Input: part model. Units: mm. Frame: model coordinates. A direction names the side the tool comes from. Coordinates: 2 decimals unless noted, no trailing zeros. Loops run counter-clockwise (first coordinate to the right, second up) from the corner with the lowest first, then second, coordinate; pieces in that order, holes last. Notation, with made-up numbers: M -20.75,8.5 L 0.25,8.5 A4 cw 0.25,15.5 Z; hole C 35.25,-12 d11. An arc over 180 degrees is marked long. Use a Markdown table: item, result. Add a question column.
1. Section B-B on z = 42.5. Output: boundary loops of the cut face in (x, y), then the cut area to 3 significant figures.
2. Section D-D on y = 7.5. Output: boundary loops of the cut face in (x, z), then the cut area to 3 significant figures.
3. Line query: L1, parallel to Z at x = -6, y = 50; L2, parallel to Y at x = -7, z = 38; L3, parallel to Y at x = -0.4, z = 38. Output: solid intervals per line, ascending. Write a range as [from, to].
4. Section C-C on x = 57. Output: boundary loops of the cut face in (y, z), then the cut area to 3 significant figures.
5. Draft query along Y for faces 1 (the cylindrical face through (-0.355, 68.506, 36.693)), 2 (the cylindrical face through (-7.145, 52.706, 39.407)), 3 (the flat face through (33, -4, 25)), 4 (the flat face through (75, 50, 1)). Return one class per face: +Y half, -Y half, draft (parallel to the pull), parting line (faces both ways), or undercut.
6. Set-up query: faces 5 (the flat face through (-4, 62.936, 13)), 6 (the flat face through (0, 49, 31)), 7 (the flat face through (-0.7, 60.4, 38)), 8 (the cylindrical face through (-7.15, 32.14, 35.85)). Return all of +Z, -Z, +X, -X, +Y, -Y with unobstructed straight access to the full face (end or side cutting, diameter ignored); none if empty.
7. Section A-A on z = 11.5. Output: boundary loops of the cut face in (x, y).
8. Pin query (flat end, axial travel): pin 1 (3 mm diameter, centred on y = 50.5, z = 38, fed in from +X); pin 2 (5 mm diameter, centred on x = 55.5, y = 37, fed in from +Z); pin 3 (8 mm diameter, centred on y = 42.1, z = 38.03, fed in from +X); pin 4 (3 mm diameter, centred on y = 58, z = 39, fed in from +X). Return the tip coordinate at first contact, or that it passes through.
Autodesk Fusion 360 part; units mm, degrees
sketch "Sketch1" plane through (0, 0, 0) normal (0, 0, 1) x (1, 0, 0)
  line L0 (0, 0) -> (140, 0)
  line L1 (140, 0) -> (140, 150)
  line L2 (140, 150) -> (0, 150)
  line L3 (0, 150) -> (0, 0)
sketch "Sketch2" plane through (0, 0, 0) normal (0, 0, 1) x (1, 0, 0)
sketch "Sketch3" plane through (0, 0, 0) normal (0, 0, 1) x (1, 0, 0)
  line L0 (0, 0) -> (0, 100)
  line L1 (0, 100) -> (75, 100)
  line L2 (75, 100) -> (75, 0)
  line L3 (75, 0) -> (0, 0)
  line L4 (75, 100) -> (75, 104)
  line L5 (75, 104) -> (-7.5, 104)
  line L6 (-7.5, 104) -> (-7.5, -4)
  line L7 (-7.5, -4) -> (75, -4)
  line L8 (75, -4) -> (75, 0)
  dimension "d4" = 75
  dimension "d5" = 4
  dimension "d6" = 82.5
  dimension "d7" = 108
  dimension "d8" = 82.5
extrude "Extrude2" add sketch "Sketch3" along normal blind 50 contours L0 L1 L3 L4 L5 L6 L7 L8
sketch "Sketch4" plane through (0, 0, 0) normal (0, 0, 1) x (1, 0, 0)
sketch "Sketch5" plane through (0, 0, 0) normal (0, 0, 1) x (1, 0, 0)
  line L0 (75, 0) -> (75, 100)
  line L1 (75, 100) -> (0, 100)
  line L2 (0, 100) -> (0, 0)
  line L3 (0, 0) -> (75, 0)
extrude "Extrude3" add sketch "Sketch5" along normal blind 1.2
sketch "Sketch6" plane through (0, 0, 0) normal (1, 0, 0) x (0, 1, 0)
  line L0 (0, 1.2) -> (100, 1.2)
  line L1 (100, 1.2) -> (100, 50)
  line L2 (100, 50) -> (0, 50)
  line L3 (0, 50) -> (0, 1.2)
sketch "Sketch7" plane through (0, 0, 0) normal (1, 0, 0) x (0, 1, 0)
  line L0 (92, -12) -> (91.9892, -11.1216)
sketch "Sketch8" plane through (0, 0, 0) normal (1, 0, 0) x (0, 1, 0)
sketch "Sketch9" plane through (0, 0, 0) normal (1, 0, 0) x (0, 1, 0)
sketch "Sketch10" plane through (0, 0, 0) normal (1, 0, 0) x (0, 1, 0)
  line L0 (0, 1.2) -> (100, 1.2)
  line L1 (100, 1.2) -> (100, 50)
  line L2 (100, 50) -> (0, 50)
  line L3 (0, 50) -> (0, 1.2)
  line L4 (37.0644, 1.2) -> (37.0644, 26)
  line L5 (37.0644, 26) -> (50, 26)
  line L6 (7, 61) -> (6, 65)
  line L7 (62.9356, 26) -> (50, 26)
  line L8 (62.9356, 1.2) -> (62.9356, 26)
sketch "Sketch11" plane through (0, 0, 0) normal (1, 0, 0) x (0, 1, 0)
  line L0 (37, 1) -> (63, 1)
extrude "Extrude4" cut sketch "Sketch10" against normal blind 16 contours L0 L4 L5 L7 L8
sketch "Sketch12" plane through (0, 0, 0) normal (1, 0, 0) x (0, 1, 0)
sketch "Sketch19" plane through (-7.5, 0, 0) normal (-1, 0, 0) x (0, -1, 0)
  line L0 (-62.9356, 1.2) -> (-62.9356, 26)
  line L1 (-62.9356, 26) -> (-37.0644, 26)
  line L2 (-37.0644, 26) -> (-37.0644, 1.2)
  line L3 (-37.0644, 1.2) -> (-62.9356, 1.2)
  line L4 (-104, 0) -> (4, 0)
  line L5 (4, 0) -> (4, 50)
  line L6 (4, 50) -> (-104, 50)
  line L7 (-104, 50) -> (-104, 0)
  line L8 (-50, 26) -> (-50, 50)
  circle A0 centre (-50, 38) radius 3.05
  line L9 (-53.0499, 38.0261) -> (-54.8499, 38.0261)
  circle A1 centre (-57.8999, 38.0261) radius 3.05
  line L10 (-60.9495, 37.9796) -> (-62.7495, 37.9796)
  circle A2 centre (-65.7995, 37.9942) radius 3.05
  circle A3 centre (-34.2005, 37.9942) radius 3.05
  circle A4 centre (-42.1001, 38.0261) radius 3.05
  line L11 (-46.9501, 38.0261) -> (-45.1501, 38.0261)
  line L12 (-39.0505, 37.9796) -> (-37.2505, 37.9796)
  circle A5 centre (-50, 38) radius 2.35
  circle A6 centre (-65.7995, 37.9942) radius 2.35
  circle A7 centre (-57.8999, 38.0261) radius 2.35
  circle A8 centre (-42.1001, 38.0261) radius 2.35
  circle A9 centre (-34.2005, 37.9942) radius 2.35
  dimension "d35" = 6.1
  dimension "d36" = 1.8
  dimension "d37" = 6.1
  dimension "d38" = 1.8
  dimension "d39" = 6.1
  dimension "d40" = 4.7
  dimension "d41" = 4.7
  dimension "d42" = 4.7
  dimension "d43" = 4.7
  dimension "d44" = 4.7
sketch "Sketch13" plane through (-7.5, 0, 0) normal (-1, 0, 0) x (0, -1, 0)
  line L0 (-62.9356, 1.2) -> (-62.9356, 26)
  line L1 (-62.9356, 26) -> (-37.0644, 26)
  line L2 (-37.0644, 26) -> (-37.0644, 1.2)
  line L3 (-37.0644, 1.2) -> (-62.9356, 1.2)
  line L4 (-104, 0) -> (4, 0)
  line L5 (4, 0) -> (4, 50)
  line L6 (4, 50) -> (-104, 50)
  line L7 (-104, 50) -> (-104, 0)
sketch "Sketch14" plane through (-7.5, 50, 25) normal (-1, 0, 0) x (0, -1, 0)
  line L0 (0.0006, 25) -> (0.0006, 1)
  line L1 (-12.9356, 1) -> (12.9356, 1)
  line L2 (54, 25) -> (-54, 25)
  circle A0 centre (0.0006, 13) radius 3.05
  circle A1 centre (0.0006, 13) radius 2.35
  dimension "d18" = 6.1
  dimension "d19" = 4.7
sketch "Sketch15" plane through (-7.5, 50, 25) normal (-1, 0, 0) x (0, -1, 0)
sketch "Sketch16" plane through (-7.5, 0, 0) normal (-1, 0, 0) x (0, -1, 0)
  line L0 (-53.0494, 38) -> (-54.8494, 38)
  circle A0 centre (-57.8994, 38) radius 3.05
  circle A1 centre (-57.8994, 38) radius 2.35
  circle A2 centre (-49.9994, 38) radius 3.05
  line L1 (-60.9494, 38) -> (-62.7494, 38)
  circle A3 centre (-65.8, 38.1) radius 3.05
  circle A4 centre (-65.8, 38.1) radius 2.35
  line L2 (-49.9994, 50) -> (-49.9994, 26)
  circle A5 centre (-42.0994, 38) radius 2.35
  circle A6 centre (-42.0994, 38) radius 3.05
  circle A7 centre (-34.1988, 38.1) radius 2.35
  circle A8 centre (-34.1988, 38.1) radius 3.05
  line L3 (-39.0494, 38) -> (-37.2494, 38)
  line L4 (-46.9494, 38) -> (-45.1494, 38)
  dimension "d24" = 1.8
  dimension "d25" = 6.1
  dimension "d26" = 4.7
  dimension "d27" = 1.8
  dimension "d28" = 6.1
  dimension "d29" = 4.7
extrude "Extrude5" cut sketch "Sketch16" against normal blind 19 contours A4
sketch "Sketch18" plane through (-7.5, 50, 25) normal (-1, 0, 0) x (0, -1, 0)
sketch "Sketch17" plane through (-7.5, 0, 0) normal (-1, 0, 0) x (0, -1, 0)
extrude "Extrude6" cut sketch "Sketch14" against normal blind 7 contours L0 A1 picked at (0.839, 13.6628)
hole "Hole1" at (-7.5, 57.8999, 38.0261) direction (1, 0, 0) diameter 4.7 depth 8 tip angle 180
sketch "Sketch20" plane through (-7.5, 0, 0) normal (-1, 0, 0) x (0, -1, 0)
sketch "Sketch21" plane through (-7.5, 0, 0) normal (-1, 0, 0) x (0, -1, 0)
  line L0 (-50, 50) -> (-50, 26)
  circle A0 centre (-50, 38) radius 3.05
  circle A1 centre (-57.8999, 38.0261) radius 3.05
  circle A2 centre (-57.8999, 38.0261) radius 2.35
  circle A3 centre (-65.8, 38.1) radius 2.9921
  circle A4 centre (-65.8, 38.1) radius 2.35
  circle A5 centre (-50, 38) radius 2.35
  dimension "d48" = 6.1
  dimension "d49" = 6.1
  dimension "d50" = 4.7
hole "Hole2" at (-7.5, 50, 38) direction (1, 0, 0) diameter 4.7 depth 8 tip angle 180
sketch "Sketch22" plane through (-7.5, 0, 0) normal (-1, 0, 0) x (0, -1, 0)
  line L0 (-50, 50) -> (-50, 26)
  circle A0 centre (-65.8, 38.1) radius 2.35
  circle A1 centre (-65.8, 38.1) radius 2.35
  circle A2 centre (-34.2, 38.1) radius 2.35
  dimension "d54" = 4.7
hole "Hole3" at (-7.5, 34.2, 38.1) direction (1, 0, 0) diameter 4.7 depth 8 tip angle 180
sketch "Sketch23" plane through (-7.5, 0, 0) normal (-1, 0, 0) x (0, -1, 0)
  circle A0 centre (-57.8999, 38.0261) radius 2.35
  circle A1 centre (-57.8999, 38.0261) radius 2.35
  line L0 (-50, 50) -> (-50, 26)
  circle A2 centre (-42.1001, 38.0261) radius 2.35
  dimension "d58" = 4.7
hole "Hole4" at (-7.5, 42.1001, 38.0261) direction (1, 0, 0) diameter 4.7 depth 8 tip angle 180
sketch "Sketch24" plane through (-7.5, 0, 0) normal (-1, 0, 0) x (0, -1, 0)
  circle A0 centre (-65.8, 38.1) radius 3.05
  circle A1 centre (-65.8, 38.1) radius 2.35
  dimension "d62" = 6.1
sketch "Sketch25" plane through (-7.5, 0, 0) normal (-1, 0, 0) x (0, -1, 0)
  circle A0 centre (-65.8, 38.1) radius 3.05
  circle A1 centre (-65.8, 38.1) radius 2.35
  dimension "d66" = 6.1
sketch "Sketch26" plane through (-7.5, 0, 0) normal (-1, 0, 0) x (0, -1, 0)
  circle A0 centre (-65.8, 38.1) radius 3.05
  circle A1 centre (-65.8, 38.1) radius 2.35
  dimension "d70" = 6.1
sketch "Sketch27" plane through (-7.5, 0, 0) normal (-1, 0, 0) x (0, -1, 0)
  circle A0 centre (-65.8, 38.1) radius 3.05
  circle A1 centre (-65.8, 38.1) radius 2.35
  dimension "d74" = 6.1
hole "Hole8" at (-7.5, 65.8, 38.1) direction (1, 0, 0) diameter 6.1 depth 0.7 tip angle 180
sketch "Sketch28" plane through (-7.5, 0, 0) normal (-1, 0, 0) x (0, -1, 0)
  circle A0 centre (-58, 38) radius 3.05
  dimension "d78" = 6.1
sketch "Sketch29" plane through (-7.5, 0, 0) normal (-1, 0, 0) x (0, -1, 0)
  circle A0 centre (-57.8999, 38.0261) radius 3.05
  circle A1 centre (-57.8999, 38.0261) radius 2.35
  dimension "d82" = 6.1
hole "Hole10" at (-7.5, 57.8999, 38.0261) direction (1, 0, 0) diameter 6.1 depth 0.7 tip angle 180
sketch "Sketch30" plane through (-7.5, 0, 0) normal (-1, 0, 0) x (0, -1, 0)
  circle A0 centre (-50, 38) radius 3.05
  dimension "d86" = 6.1
hole "Hole11" at (-7.5, 50, 38) direction (1, 0, 0) diameter 6.1 depth 0.7 tip angle 180
sketch "Sketch31" plane through (-7.5, 0, 0) normal (-1, 0, 0) x (0, -1, 0)
  circle A0 centre (-42.1001, 38.0261) radius 3.05
  circle A1 centre (-42.1001, 38.0261) radius 2.35
  dimension "d90" = 6.1
hole "Hole12" at (-7.5, 42.1001, 38.0261) direction (1, 0, 0) diameter 6.1 depth 0.7 tip angle 180
sketch "Sketch32" plane through (-7.5, 0, 0) normal (-1, 0, 0) x (0, -1, 0)
  circle A0 centre (-34.2, 38.1) radius 3.05
  circle A1 centre (-34.2, 38.1) radius 2.35
  dimension "d94" = 6.1
hole "Hole13" at (-7.5, 34.2, 38.1) direction (1, 0, 0) diameter 6.1 depth 0.7 tip angle 180
sketch "Sketch33" plane through (0, 0, 0) normal (1, 0, 0) x (0, 1, 0)
  circle A0 centre (34.2, 38.1) radius 3.05
  circle A1 centre (34.2, 38.1) radius 2.35
  dimension "d98" = 6.1
hole "Hole14" at (0, 34.2, 38.1) direction (-1, 0, 0) diameter 6.1 depth 0.7 tip angle 180
sketch "Sketch34" plane through (0, 0, 0) normal (1, 0, 0) x (0, 1, 0)
  circle A0 centre (42.1001, 38.0261) radius 3.05
  circle A1 centre (42.1001, 38.0261) radius 2.35
  dimension "d102" = 6.1
hole "Hole15" at (0, 42.1001, 38.0261) direction (-1, 0, 0) diameter 6.1 depth 0.7 tip angle 180
sketch "Sketch35" plane through (0, 0, 0) normal (1, 0, 0) x (0, 1, 0)
  circle A0 centre (50, 38) radius 3.05
  dimension "d107" = 6.1
hole "Hole16" at (0, 50, 38) direction (-1, 0, 0) diameter 6.1 depth 0.7 tip angle 180
sketch "Sketch36" plane through (0, 0, 0) normal (1, 0, 0) x (0, 1, 0)
  circle A0 centre (57.8999, 38.0261) radius 3.05
  circle A1 centre (57.8999, 38.0261) radius 2.35
  dimension "d111" = 6.1
hole "Hole17" at (0, 57.8999, 38.0261) direction (-1, 0, 0) diameter 6.1 depth 0.7 tip angle 180
sketch "Sketch37" plane through (0, 0, 0) normal (1, 0, 0) x (0, 1, 0)
  circle A0 centre (65.8, 38.1) radius 3.05
  circle A1 centre (65.8, 38.1) radius 2.35
  dimension "d115" = 6.1
hole "Hole18" at (0, 65.8, 38.1) direction (-1, 0, 0) diameter 6.1 depth 0.7 tip angle 180
hole "Hole9" at (-7.5, 58, 38) direction (1, 0, 0) diameter 6.1 depth 0.7 tip angle 180
hole "Hole7" at (-7.5, 65.8, 38.1) direction (1, 0, 0) diameter 6.1 depth 1 tip angle 180
hole "Hole6" at (-7.5, 65.8, 38.1) direction (1, 0, 0) diameter 6.1 depth 1.2 tip angle 180
hole "Hole5" at (-7.5, 65.8, 38.1) direction (1, 0, 0) diameter 6.1 depth 0.1 tip angle 180
Answers below:
| question | item | result |
|---|---|---|
| 1 | outline | M -7.5,-4 L 75,-4 L 75,0 L 0,0 L 0,100 L 75,100 L 75,104 L -7.5,104 Z |
| 1 | area | 1,410 mm² |
| 2 | outline | M -7.5,0 L 75,0 L 75,1.2 L 0,1.2 L 0,50 L -7.5,50 Z |
| 2 | area | 465 mm² |
| 3 | L1 | z = [0, 1.2], [26, 35.65], [40.35, 50] |
| 3 | L2 | y = [-4, 31.15], [37.25, 39.05], [45.15, 46.95], [53.05, 54.85], [61.05, 62.75], [68.85, 104] |
| 3 | L3 | y = [-4, 31.15], [37.25, 39.05], [45.15, 46.95], [53.05, 54.85], [60.95, 62.75], [68.85, 104] |
| 4 | outline | M -4,0 L 104,0 L 104,50 L 100,50 L 100,1.2 L 0,1.2 L 0,50 L -4,50 Z |
| 4 | area | 520 mm² |
| 5 | face 1 | undercut |
| 5 | face 2 | undercut |
| 5 | face 3 | -Y half |
| 5 | face 4 | draft |
| 6 | face 5 | +X, -X |
| 6 | face 6 | +Z, +X |
| 6 | face 7 | +X |
| 6 | face 8 | -X |
| 7 | outline | M -7.5,-4 L 75,-4 L 75,0 L 0,0 L 0,37.06 L -7.5,37.06 Z; M -7.5,62.94 L 0,62.94 L 0,100 L 75,100 L 75,104 L -7.5,104 Z |
| 8 | pin 1 | passes through |
| 8 | pin 2 | stops at z = 1.2 |
| 8 | pin 3 | stops at x = 0 |
| 8 | pin 4 | stops at x = -0.7 |
